Could you check a few things on this model? Use its own coordinates, in mm. A direction names the side the tool comes from. Coordinates: 2 decimals unless noted, no trailing zeros. Order: outer loops, then holes, each group sorted by start corner. A loop starts at its lowest first (then second) coordinate and runs counter-clockwise, first axis right, second up. Notation, with made-up numbers: M 9,68 L 48,68 A12 ccw 48,72 Z; hole C 72,67 d9. An arc over 180 degrees is marked long. Put each result on its own line as item: value. Start each with the question number.
Autodesk Inventor part; units mm, degrees
ref_plane "YZ Plane" through (0, 0, 0) normal (1, 0, 0) x (0, 1, 0)
ref_plane "XZ Plane" through (0, 0, 0) normal (0, 1, 0) x (-1, 0, 0)
ref_plane "XY Plane" through (0, 0, 0) normal (0, 0, 1) x (1, 0, 0)
sketch "Sketch1" plane through (0, 0, 0) normal (0, 0, 1) x (1, 0, 0)
  circle A0 centre (0, 0) radius 38.1
  dimension "d2" = 76.2
extrude "Extrusion1" add sketch "Sketch1" along normal mid plane 6.35
sketch "Sketch2" plane through (0, 0, 3.175) normal (0, 0, 1) x (1, 0, 0)
  circle A0 centre (0, 0) radius 38.1
  point P0 (0, 28.575)
  dimension "d3" = 0
  dimension "d4" = 28.575
hole "Mounting Hole" at (0, 28.575, 3.175) direction (0, 0, -1) diameter 6.35 end through all
pattern_circular "Circular Pattern1" count 4 over 360 about axis through (0, 0, 0) along (0, 0, 1) of "Mounting Hole"
sketch "Sketch5" plane through (0, 0, -3.175) normal (0, 0, -1) x (-1, 0, 0)
  circle A0 centre (0, 0) radius 38.1
  circle A1 centre (0, 0) radius 14.9225
  dimension "d27" = 29.845
extrude "Extrusion4" add sketch "Sketch5" along normal blind 25.4 draft -5 contours A1
sketch "Sketch6" plane through (0, 0, -28.575) normal (0, 0, -1) x (-1, 0, 0)
  circle A0 centre (0, 0) radius 12.7003
  arc A1 (2.3812, -7.6374) -> (-2.3813, -7.6374) centre (0, 0) ccw
  line L0 (-2.3813, -7.6374) -> (-2.3812, -10.3188)
  line L1 (-2.3812, -10.3188) -> (2.3813, -10.3188)
  line L2 (2.3813, -10.3188) -> (2.3812, -7.6374)
  dimension "d31" = 16
  dimension "d32" = 4.7625
  dimension "d33" = 10.3187
extrude "Extrusion5" cut sketch "Sketch6" against normal blind 28.575 contours L2 L1 L0 A1
sketch "Sketch7" plane through (0, 0, 0) normal (0, 0, -1) x (-1, 0, 0)
  arc A0 (2.3812, -7.6374) -> (-2.3813, -7.6374) centre (0, 0) ccw
  point P0 (0, 0)
hole "Hole2" at (0, 0, 0) direction (0, 0, 1) diameter 9.525 end through all
sketch "Sketch3" plane through (0, 0, 3.175) normal (0, 0, 1) x (1, 0, 0)
  circle A0 centre (0, 0) radius 38.1
  circle A1 centre (0, 0) radius 15.875
  dimension "d15" = 31.75
extrude "Extrusion2" add sketch "Sketch3" along normal blind 12.7 contours A1
sketch "Sketch8" plane through (0, 0, 15.875) normal (0, 0, 1) x (1, 0, 0)
  circle A0 centre (0, 0) radius 15.875
hole "Hole3" at (0, 0, 15.875) direction (0, 0, -1) diameter 16.2 depth 14.986
sketch "Sketch4" plane through (0, 0, 15.875) normal (0, 0, 1) x (1, 0, 0)
  circle A0 centre (0, 0) radius 15.875
  circle A1 centre (0, 0) radius 8.1
  arc A2 (-6.1113, 9.1462) -> (-4.9718, 5.6692) centre (3.287, 10.3011) ccw
  arc A3 (-4.9718, 5.6692) -> (-5.6692, 4.9718) centre (0, 0) ccw
  arc A4 (-5.6692, 4.9718) -> (-9.1462, 6.1113) centre (-10.3011, -3.287) ccw
  arc A5 (-9.1462, 6.1113) -> (-9.8656, 4.8652) centre (0, 0) ccw
  arc A6 (-9.8656, 4.8652) -> (-7.1403, 2.4238) centre (-2.3039, 10.5645) ccw
  arc A7 (-7.1403, 2.4238) -> (-7.3956, 1.4711) centre (0, 0) ccw
  arc A8 (-7.3956, 1.4711) -> (-10.9764, 0.7194) centre (-7.2775, -7.9972) ccw
  arc A9 (-10.9764, 0.7194) -> (-10.9764, -0.7194) centre (0, 0) ccw
  arc A10 (-10.9764, -0.7194) -> (-7.3956, -1.4711) centre (-7.2775, 7.9972) ccw
  arc A11 (-7.3956, -1.4711) -> (-7.1403, -2.4238) centre (0, 0) ccw
  arc A12 (-7.1403, -2.4238) -> (-9.8656, -4.8652) centre (-2.3039, -10.5645) ccw
  arc A13 (-9.8656, -4.8652) -> (-9.1462, -6.1113) centre (0, 0) ccw
  arc A14 (-9.1462, -6.1113) -> (-5.6692, -4.9718) centre (-10.3011, 3.287) ccw
  arc A15 (-5.6692, -4.9718) -> (-4.9718, -5.6692) centre (0, 0) ccw
  arc A16 (-4.9718, -5.6692) -> (-6.1113, -9.1462) centre (3.287, -10.3011) ccw
  arc A17 (-6.1113, -9.1462) -> (-4.8652, -9.8656) centre (0, 0) ccw
  arc A18 (-4.8652, -9.8656) -> (-2.4238, -7.1403) centre (-10.5645, -2.3039) ccw
  arc A19 (-2.4238, -7.1403) -> (-1.4711, -7.3956) centre (0, 0) ccw
  arc A20 (-1.4711, -7.3956) -> (-0.7194, -10.9764) centre (7.9972, -7.2775) ccw
  arc A21 (-0.7194, -10.9764) -> (0.7194, -10.9764) centre (0, 0) ccw
  arc A22 (0.7194, -10.9764) -> (1.4711, -7.3956) centre (-7.9972, -7.2775) ccw
  arc A23 (1.4711, -7.3956) -> (2.4238, -7.1403) centre (0, 0) ccw
  arc A24 (2.4238, -7.1403) -> (4.8652, -9.8656) centre (10.5645, -2.3039) ccw
  arc A25 (4.8652, -9.8656) -> (6.1113, -9.1462) centre (0, 0) ccw
  arc A26 (6.1113, -9.1462) -> (4.9718, -5.6692) centre (-3.287, -10.3011) ccw
  arc A27 (4.9718, -5.6692) -> (5.6692, -4.9718) centre (0, 0) ccw
  arc A28 (5.6692, -4.9718) -> (9.1462, -6.1113) centre (10.3011, 3.287) ccw
  arc A29 (9.1462, -6.1113) -> (9.8656, -4.8652) centre (0, 0) ccw
  arc A30 (9.8656, -4.8652) -> (7.1403, -2.4238) centre (2.3039, -10.5645) ccw
  arc A31 (7.1403, -2.4238) -> (7.3956, -1.4711) centre (0, 0) ccw
  arc A32 (7.3956, -1.4711) -> (10.9764, -0.7194) centre (7.2775, 7.9972) ccw
  arc A33 (10.9764, -0.7194) -> (10.9764, 0.7194) centre (0, 0) ccw
  arc A34 (10.9764, 0.7194) -> (7.3956, 1.4711) centre (7.2775, -7.9972) ccw
  arc A35 (7.3956, 1.4711) -> (7.1403, 2.4238) centre (0, 0) ccw
  arc A36 (7.1403, 2.4238) -> (9.8656, 4.8652) centre (2.3039, 10.5645) ccw
  arc A37 (9.8656, 4.8652) -> (9.1462, 6.1113) centre (0, 0) ccw
  arc A38 (9.1462, 6.1113) -> (5.6692, 4.9718) centre (10.3011, -3.287) ccw
  arc A39 (5.6692, 4.9718) -> (4.9718, 5.6692) centre (0, 0) ccw
  arc A40 (4.9718, 5.6692) -> (6.1113, 9.1462) centre (-3.287, 10.3011) ccw
  arc A41 (6.1113, 9.1462) -> (4.8652, 9.8656) centre (0, 0) ccw
  arc A42 (4.8652, 9.8656) -> (2.4238, 7.1403) centre (10.5645, 2.3039) ccw
  arc A43 (2.4238, 7.1403) -> (1.4711, 7.3956) centre (0, 0) ccw
  arc A44 (1.4711, 7.3956) -> (0.7194, 10.9764) centre (-7.9972, 7.2775) ccw
  arc A45 (0.7194, 10.9764) -> (-0.7194, 10.9764) centre (0, 0) ccw
  arc A46 (-0.7194, 10.9764) -> (-1.4711, 7.3956) centre (7.9972, 7.2775) ccw
  arc A47 (-1.4711, 7.3956) -> (-2.4238, 7.1403) centre (0, 0) ccw
  arc A48 (-2.4238, 7.1403) -> (-4.8652, 9.8656) centre (-10.5645, 2.3039) ccw
  arc A49 (-4.8652, 9.8656) -> (-6.1113, 9.1462) centre (0, 0) ccw
extrude "Extrusion3" cut sketch "Sketch4" against normal up to surface (14.986 mm away) contours A1 A32 A31 A30 A28 A27 A26 A24 A23 A22 A20 A19 A18 A16 A15 A14 A12 A11 A10 A8 A7 A6 A4 A3 A2 A48 A47 A46 A44 A43 A42 A40 A39 A38 A36 A35 A34 | A1 A34 A33 A32 | A1 A38 A37 A36 | A30 A29 A28 A1 | A1 A42 A41 A40 | A26 A25 A24 A1 | A1 A46 A45 A44 | A22 A21 A20 A1 | A1 A2 A49 A48 | A18 A17 A16 A1 | A1 A6 A5 A4 | A14 A13 A12 A1 | A1 A10 A9 A8
fillet "Fillet1" radius 0.508 2 edges at (14.9225, 0, -3.175) (-15.875, 0, 3.175)
properties part number "Keyang-12" material "ABS Plastic"
Item 1: If we section it at C-C on z = -11.5: Write out the boundary of the cut face in (x, y), then the cut area to 3 significant figures.
Item 2: If we section it at A-A on z = -20: Write out the boundary of the cut face in (x, y).
Item 3: If we section it at B-B on y = 19: Write out the boundary of the cut face in (x, z) (3 decimals).
Item 4: I need wall thicknesses on probe 1 along Z at (x, y) = (-22, 23) (3 decimals); probe 2 along X at (y, z) = (1.5, -11); probe 3 along Y at (x, z) = (7, -9). Which ranges of each line are inside material? Lowest first, please.
Item 5: For pin 1 Ø4 at (x, y) = (4, 27) entering from -Z (3 decimals); pin 2 Ø5 at (x, y) = (-28.5, -6.5) entering from +Z (3 decimals); pin 3 Ø1 at (x, y) = (-9, -5) entering from +Z; pin 4 Ø13 at (x, y) = (0.5, -4.5) entering from -Z (3 decimals), each with a flat end and sliding along its axis, tell me the tip position at first contact or that it passes through.
Item 6: If we mould it in two halves opening along Y, with no side actions, what happens to faces 1 (the flat face through (-8.3, 0.2, -28.575)), 2 (the cylindrical face through (2.9, -3.78, 0.45))? For each: released by +Y, released by -Y, zero draft, split by the parting line, or undercut.
Item 7: For faces 3 (the cylindrical face through (-1.932, -31.095, -0.044)), 4 (the flat face through (16, 1, -3.175)), 5 (the cylindrical face through (1.212, 9.482, 8.487)), which set-ups out of +Z, -Z, +X, -X, +Y, -Y let a thin tool reach every point of the face, with its end or its side?
Geometry check:
1. outline: C 0,0 d28.39; hole M -2.38,-10.32 L 2.38,-10.32 L 2.38,-7.64 A8 ccw long -2.38,-7.64 Z
1. area: 420 mm²
2. outline: C 0,0 d26.9; hole M -2.38,-10.32 L 2.38,-10.32 L 2.38,-7.64 A8 ccw long -2.38,-7.64 Z
3. outline: M -33.024,-3.175 L 33.024,-3.175 L 33.024,3.175 L -33.024,3.175 Z
4. probe 1: z = -3.175 to 3.175
4. probe 2: x = -14.16 to -7.86, 7.86 to 14.16
4. probe 3: y = -12.6 to -3.87, 3.87 to 12.6
5. pin 1: stops at z = -3.175
5. pin 2: stops at z = 3.175
5. pin 3: stops at z = 0.89
5. pin 4: stops at z = -28.575
6. face 1: zero draft
6. face 2: undercut
7. face 3: +Z, -Z
7. face 4: -Z
7. face 5: +Z
